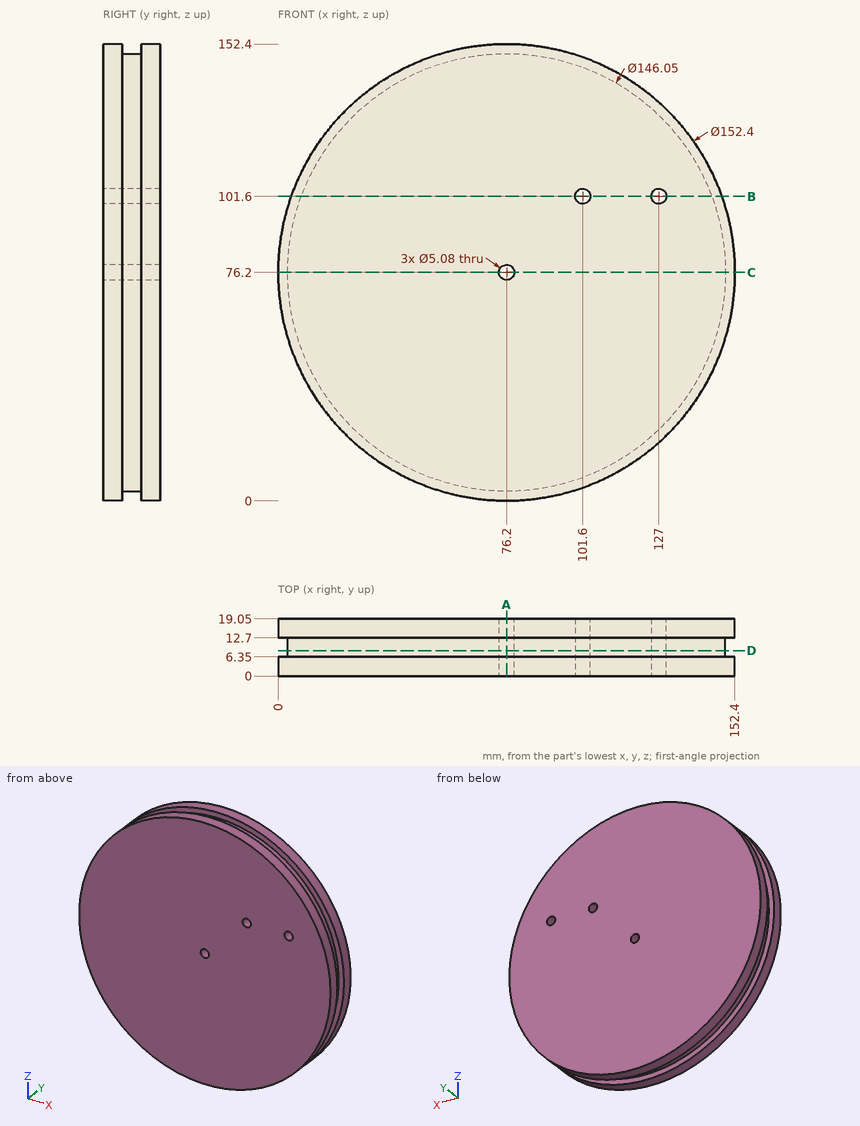
Study the drawing (mm; zero at the part's minimum x, y, z) and answer. Coordinates: 2 decimals unless noted, no trailing zeros. Loops run counter-clockwise (first coordinate to the right, second up) from the corner with the lowest first, then second, coordinate; pieces in that order, holes last. Notation, with made-up numbers: (20, 44.5) -> (24, 44.5) arc R8 cw to (24, 49.5) -> close; hole circle Ø2 at (9.25, -22.5). An arc over 180 degrees is marked (long way). Write item = value, one per line. Start each with the question number.
1) The part is cut by section C-C, the plane z = 76.2. Determine the outline of the cut face in (x, y) (3 decimals).
2) Find the intervals of material crossed by L1, parallel to X at y = 2.5, z = 103; L2, parallel to Z at x = 76.2, y = 12 (3 decimals); L3, parallel to Z at x = 101.6, y = 8.5, in increasing order. Write a range as from..to.
3) The part is cut by section B-B, the plane z = 101.6. Determine the outline of the cut face in (x, y), plus the area to 3 significant figures.
4) Given P1, Ø8, axis at x = 30.5, y = 14.5, coming from the +Z side; P2, Ø8, axis at x = 54, z = 37.5, coming from the -Y side; P3, Ø4.5, axis at x = 127, z = 101.6, coming from the +Y side; P4, Ø8, axis at y = 17, z = 39.5, coming from the -X side, each flat-ended and moving along its own axis, determine where each tip first touches the part or whether it passes through.
5) The part is cut by section D-D, the plane y = 8.5. Determine the outline of the cut face in (x, z) (3 decimals), plus the area to 3 significant figures.
6) The part is cut by section A-A, the plane x = 76.2. Determine the outline of the cut face in (y, z) (3 decimals), plus the area to 3 significant figures.
Result:
q1.outline = (0, 0) -> (73.66, 0) -> (73.66, 19.05) -> (0, 19.05) -> (0, 12.7) -> (3.175, 12.7) -> (3.175, 6.35) -> (0, 6.35) -> close; (78.74, 0) -> (152.4, 0) -> (152.4, 6.35) -> (149.225, 6.35) -> (149.225, 12.7) -> (152.4, 12.7) -> (152.4, 19.05) -> (78.74, 19.05) -> close
q2.L1 = 4.87..99.48, 103.72..124.88, 129.12..147.53
q2.L2 = 3.175..73.66, 78.74..149.225
q2.L3 = 7.73..99.06, 104.14..144.67
q3.outline = (4.36, 0) -> (99.06, 0) -> (99.06, 19.05) -> (4.36, 19.05) -> (4.36, 12.7) -> (7.73, 12.7) -> (7.73, 6.35) -> (4.36, 6.35) -> close; (104.14, 0) -> (124.46, 0) -> (124.46, 19.05) -> (104.14, 19.05) -> close; (129.54, 0) -> (148.04, 0) -> (148.04, 6.35) -> (144.67, 6.35) -> (144.67, 12.7) -> (148.04, 12.7) -> (148.04, 19.05) -> (129.54, 19.05) -> close
q3.area = 2,500 mm²
q4.P1 = 139.98
q4.P2 = 0
q4.P3 = through
q4.P4 = 7.37
q5.outline = circle Ø146.05 at (76.2, 76.2); hole circle Ø5.08 at (76.2, 76.2); hole circle Ø5.08 at (101.6, 101.6); hole circle Ø5.08 at (127, 101.6)
q5.area = 16,700 mm²
q6.outline = (0, 0) -> (6.35, 0) -> (6.35, 3.175) -> (12.7, 3.175) -> (12.7, 0) -> (19.05, 0) -> (19.05, 73.66) -> (0, 73.66) -> close; (0, 78.74) -> (19.05, 78.74) -> (19.05, 152.4) -> (12.7, 152.4) -> (12.7, 149.225) -> (6.35, 149.225) -> (6.35, 152.4) -> (0, 152.4) -> close
q6.area = 2,770 mm²
